from build123d import *

# Parameters (mm, degrees)
SKETCH1_W           = 37
SKETCH1_H           = 6
SKETCH1_R           = 3.2
BOSS_EXTRUDE1_DEPTH = 20
CUT_EXTRUDE2_START  = -6
SKETCH2_R           = 8.2
SKETCH2_R_2         = 1.7
CUT_EXTRUDE2_DEPTH  = 7
FILLET1_R           = 5


with BuildPart() as part:
    # Sketch1 → Boss-Extrude1 (new body, symmetric)
    with BuildSketch(Plane(origin=(0, 0, 0), x_dir=(1, 0, 0), z_dir=(0, 1, 0))):
        with Locations((0, 3)):
            Rectangle(SKETCH1_W, SKETCH1_H)
        with BuildLine():
            Line((18.5, 6), (18.5, 0))
            Line((18.5, 0), (25.7, 0))
            Line((25.7, 0), (30.679959839, 6))
            ThreePointArc((30.679959839, 6), (28.527038128, 17.821771321), (18.5, 11.2))
            Line((18.5, 11.2), (18.5, 6))
        make_face()
        with Locations((25.7, 11.2)):
            Circle(SKETCH1_R, mode=Mode.SUBTRACT)
        with BuildLine():
            Line((-25.7, 0), (-18.5, 0))
            Line((-18.5, 0), (-18.5, 6))
            Line((-18.5, 6), (-18.5, 11.2))
            ThreePointArc((-18.5, 11.2), (-28.527038128, 17.821771321), (-30.679959839, 6))
            Line((-30.679959839, 6), (-25.7, 0))
        make_face()
        with Locations((-25.7, 11.2)):
            Circle(SKETCH1_R, mode=Mode.SUBTRACT)
    extrude(amount=BOSS_EXTRUDE1_DEPTH, both=True)

    # Sketch2 → Cut-Extrude2 (cut, through all)
    with BuildSketch(Plane.XY.offset(CUT_EXTRUDE2_START)):
        Circle(SKETCH2_R)
        with Locations((0, -11.893415545)):
            Circle(SKETCH2_R_2)
        with Locations((-10.3, 5.946707773)):
            Circle(SKETCH2_R_2)
        with Locations((10.3, 5.946707773)):
            Circle(SKETCH2_R_2)
    extrude(amount=CUT_EXTRUDE2_DEPTH, mode=Mode.SUBTRACT)

    # Fillet1
    fillet1_edges = [part.edges().sort_by_distance(p)[0] for p in [
        (25.7, 0, 0),
        (-25.7, 0, 0),
    ]]
    fillet(fillet1_edges, radius=FILLET1_R)


solid = part.part
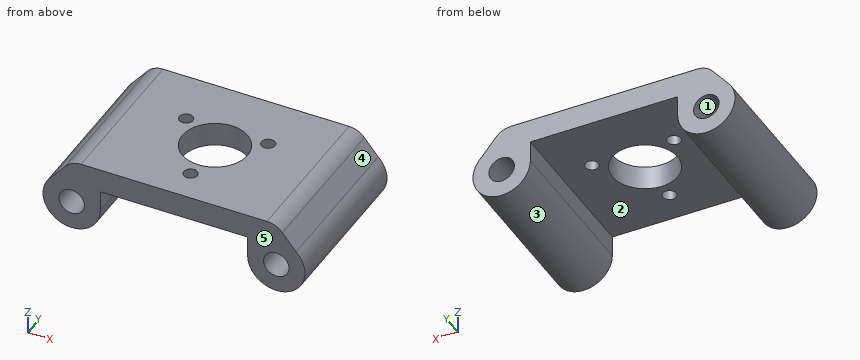
The listing builds one solid part. Answer for the finished solid, in the listing's coordinates (mm). Face numbers are marked on the shaded views. A direction names the side the tool comes from. Coordinates: 2 decimals unless noted, no trailing zeros. Write each loop counter-clockwise with the first axis right and the second up, starting at its lowest first coordinate (ties: lowest second). Pieces come first, ordered by that corner, then holes. Notation, with made-up numbers: M 0.5,-33.5 L 25.5,-33.5 A27 ccw 25.5,-12.5 Z; hole C 53.25,52 d6. An arc over 180 degrees is marked long. Use one line per item in the form item = value.
Item 1: Find the intervals of material crossed by probe 1 along Y at (x, z) = (0, -2.4); probe 2 along X at (y, z) = (-4, -11.5); probe 3 along Y at (x, z) = (-10.3, -4.3), in increasing order.
Model answer:
probe_1 = -20 to -13.59, -10.19 to -8.2, 8.2 to 20
probe_2 = -32.89 to -28.89, -22.51 to -18.51, 18.51 to 22.51, 28.89 to 32.89
probe_3 = -20 to 4.25, 7.65 to 20
Item 2: Find section B-B, the plane y = 0. Give the vertices of the cut face in (x, z), plus the area to 3 significant figures.
Model answer:
outline = M -30.68,-6 A7.2 ccw long -18.5,-11.2 L -18.5,-6 L -8.2,-6 L -8.2,0 L -23.35,0 A5 ccw -27.2,-1.81 Z; M 8.2,-6 L 18.5,-6 L 18.5,-11.2 A7.2 ccw long 30.68,-6 L 27.2,-1.81 A5 ccw 23.35,0 L 8.2,0 Z; hole C -25.7,-11.2 d6.4; hole C 25.7,-11.2 d6.4
area = 479 mm2
Item 3: Given P1, Ø5, axis at y = -4, z = -3, coming from the +X side; P2, Ø15, axis at x = 0, y = 0, coming from the -Z side; P3, Ø4, axis at y = -2.5, z = -9, coming from the -X side; P4, Ø3, axis at x = 12.5, y = -5, coming from the -Z side, each flat-ended and moving along its own axis, determine where each tip first touches the part or whether it passes through.
Model answer:
P1 = 30.26
P2 = through
P3 = -32.9
P4 = -6
Item 4: Find section D-D, the plane x = 0. Give the vertices of the cut face in (y, z).
Model answer:
outline = M -20,-6 L -13.59,-6 L -13.59,0 L -20,0 Z; M -10.19,-6 L -8.2,-6 L -8.2,0 L -10.19,0 Z; M 8.2,-6 L 20,-6 L 20,0 L 8.2,0 Z
Item 5: For the marked faces 1 and 2, determine the directions among +Z, -Z, +X, -X, +Y, -Y from which every point of the face is accessible in a straight line to the end or side of a thin tool.
Model answer:
face_1 = +Y, -Y
face_2 = -Z, +Y, -Y
Item 6: Find section A-A, the plane x = 10.3. Give the vertices of the cut face in (y, z).
Model answer:
outline = M -20,-6 L 4.25,-6 L 4.25,0 L -20,0 Z; M 7.65,-6 L 20,-6 L 20,0 L 7.65,0 Z
Item 7: The mould has two halves that part along X. Classify the marked faces 3, 4 and 5: released by +X, released by -X, zero draft, split by the parting line, or undercut.
Model answer:
face_3 = undercut
face_4 = released by +X
face_5 = zero draft
Item 8: Find section C-C, the plane y = -14.5. Give the vertices of the cut face in (x, z).
Model answer:
outline = M -30.68,-6 A7.2 ccw long -18.5,-11.2 L -18.5,-6 L 18.5,-6 L 18.5,-11.2 A7.2 ccw long 30.68,-6 L 27.2,-1.81 A5 ccw 23.35,0 L -23.35,0 A5 ccw -27.2,-1.81 Z; hole C -25.7,-11.2 d6.4; hole C 25.7,-11.2 d6.4
